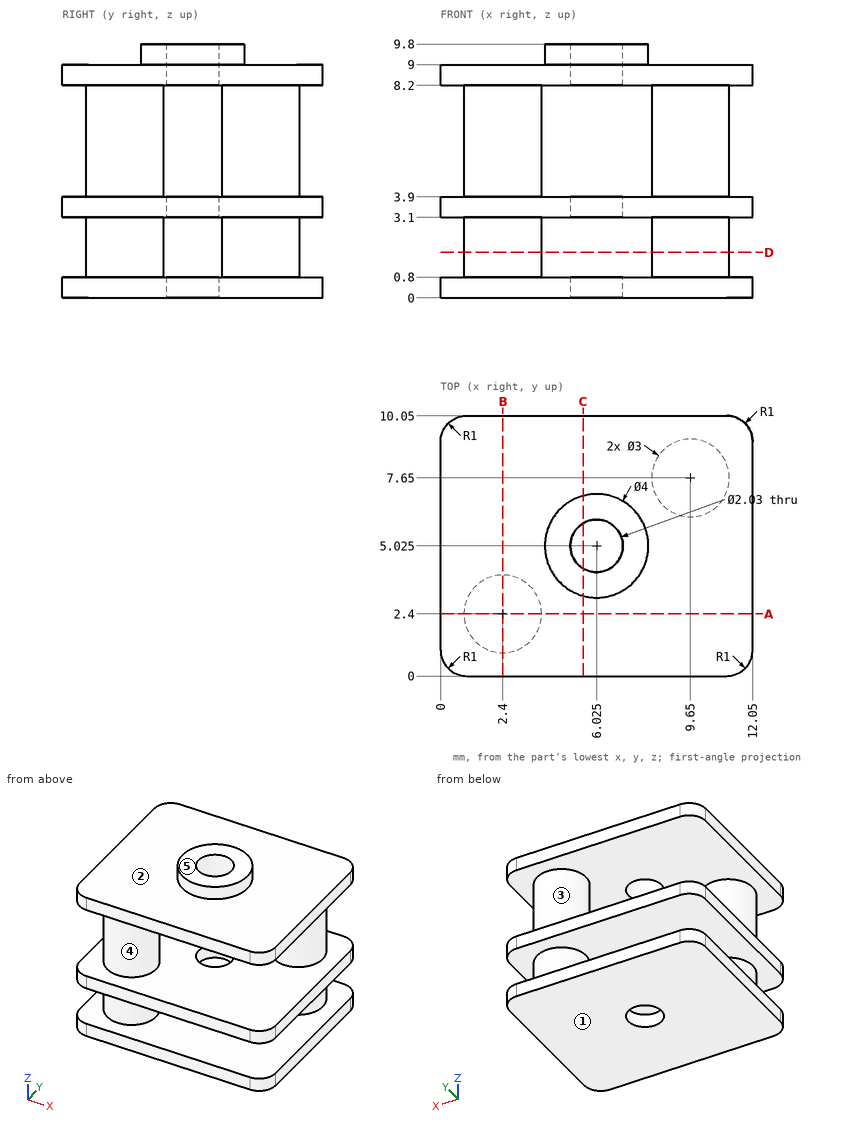
Can you work these out from the drawing? Everything is in mm from the part's minimum corner. A direction names the side the tool comes from. Round coordinates to 2 decimals unless told otherwise and drop trailing zeros. Write each loop counter-clockwise with the first axis right and the second up, starting at its lowest first coordinate (ties: lowest second). Pieces come first, ordered by that corner, then holes. Notation, with made-up numbers: (-27, 40.5) - (-11, 40.5) arc R33 ccw to (-11, 74.5) - close; hole circle Ø7 at (-21.75, -31). An arc over 180 degrees is marked (long way). Use a Markdown table: item, result.
Q1. For the marked faces 4 and 5, which set-ups out of +Z, -Z, +X, -X, +Y, -Y let a thin tool reach every point of the face, with its end or its side?
Output values:
| item | result |
|---|---|
| face 4 | none |
| face 5 | +Z, +X, -X, +Y, -Y |
Q2. For pin 1 (1.6 mm diameter, centred on x = 6.025, y = 5.025, fed in from +Z), with a flat end and sliding along its axis, tell me the tip position at first contact or that it passes through.
Output values:
| item | result |
|---|---|
| pin 1 | through |
Q3. I want a section at C-C (x = 5.5). List the corners of the cut face in (y, z) for me, plus the area to 3 significant figures.
Output values:
| item | result |
|---|---|
| outline | (0, 0) - (4.16, 0) - (4.16, 0.8) - (0, 0.8) - close; (0, 3.1) - (4.16, 3.1) - (4.16, 3.9) - (0, 3.9) - close; (0, 8.2) - (4.16, 8.2) - (4.16, 9.8) - (3.1, 9.8) - (3.1, 9) - (0, 9) - close; (5.89, 0) - (10.05, 0) - (10.05, 0.8) - (5.89, 0.8) - close; (5.89, 3.1) - (10.05, 3.1) - (10.05, 3.9) - (5.89, 3.9) - close; (5.89, 8.2) - (10.05, 8.2) - (10.05, 9) - (6.95, 9) - (6.95, 9.8) - (5.89, 9.8) - close |
| area | 21.6 mm2 |
Q4. I want a section at A-A (y = 2.4). List the corners of the cut face in (x, z) for me.
Output values:
| item | result |
|---|---|
| outline | (0, 0) - (12.05, 0) - (12.05, 0.8) - (3.9, 0.8) - (3.9, 3.1) - (12.05, 3.1) - (12.05, 3.9) - (3.9, 3.9) - (3.9, 8.2) - (12.05, 8.2) - (12.05, 9) - (0, 9) - (0, 8.2) - (0.9, 8.2) - (0.9, 3.9) - (0, 3.9) - (0, 3.1) - (0.9, 3.1) - (0.9, 0.8) - (0, 0.8) - close |
Q5. I want a section at D-D (z = 1.75). List the corners of the cut face in (x, y) for me.
Output values:
| item | result |
|---|---|
| outline | circle Ø3 at (2.4, 2.4); circle Ø3 at (9.65, 7.65) |
Q6. I want a section at B-B (x = 2.4). List the corners of the cut face in (y, z) for me, plus the area to 3 significant figures.
Output values:
| item | result |
|---|---|
| outline | (0, 0) - (10.05, 0) - (10.05, 0.8) - (3.9, 0.8) - (3.9, 3.1) - (10.05, 3.1) - (10.05, 3.9) - (3.9, 3.9) - (3.9, 8.2) - (10.05, 8.2) - (10.05, 9) - (0, 9) - (0, 8.2) - (0.9, 8.2) - (0.9, 3.9) - (0, 3.9) - (0, 3.1) - (0.9, 3.1) - (0.9, 0.8) - (0, 0.8) - close |
| area | 43.9 mm2 |
Q7. Please list where these lines run through material, in increasing order: L1, parallel to Z at x = 6.5, y = 3.5; L2, parallel to Z at x = 0.75, y = 2.5; L3, parallel to Z at x = 3.5, y = 2.
Output values:
| item | result |
|---|---|
| L1 | 0 to 0.8, 3.1 to 3.9, 8.2 to 9.8 |
| L2 | 0 to 0.8, 3.1 to 3.9, 8.2 to 9 |
| L3 | 0 to 9 |
Q8. Thinking about a two-plate mould opening in Z: for the marked faces 1, 2 and 3, which applies, released by +Z, released by -Z, zero draft, split by the parting line, or undercut?
Output values:
| item | result |
|---|---|
| face 1 | released by -Z |
| face 2 | released by +Z |
| face 3 | undercut |
